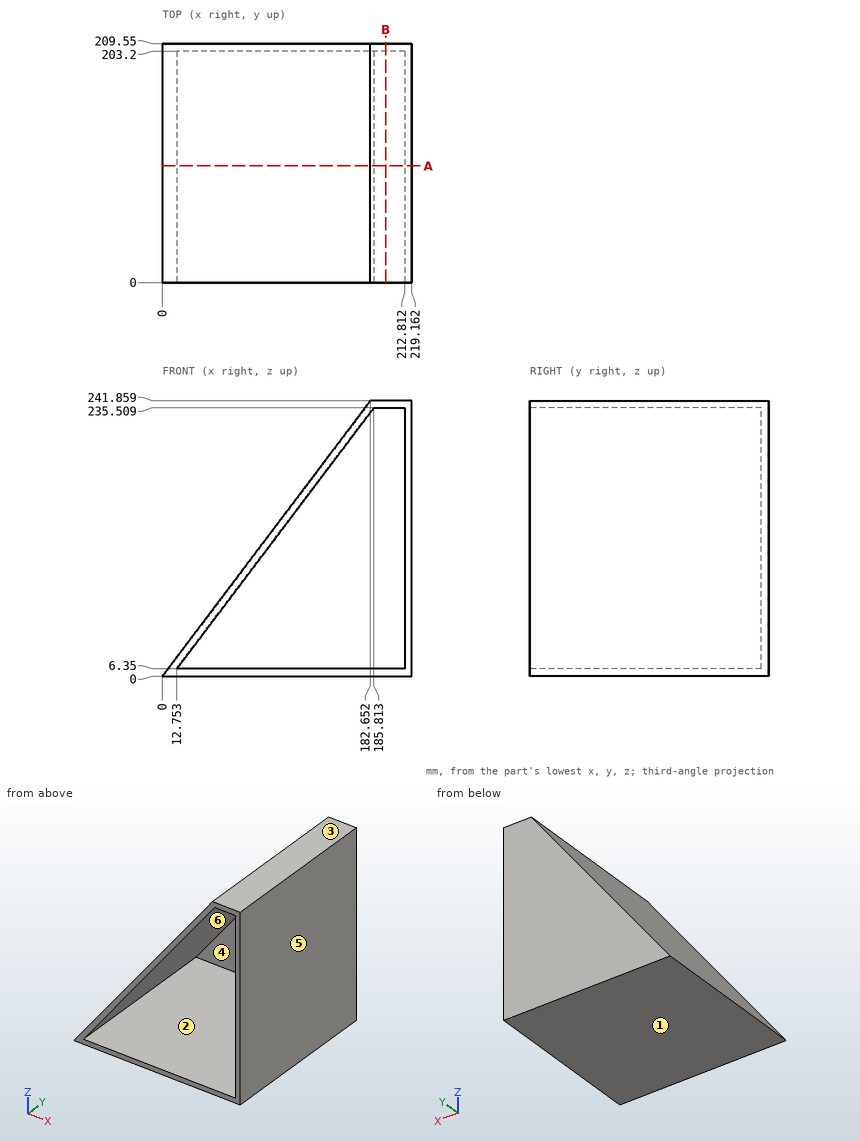
Geometry: see drawing. Coordinates: mm, zero at the bounding-box minimum. A direction names the side the tool comes from. Round coordinates to 2 decimals unless told otherwise and drop trailing zeros. Loops run counter-clockwise (first coordinate to the right, second up) from the corner with the lowest first, then second, coordinate; pieces in that order, holes last.
(1) Pull-direction query (X, two-part tool) for the marked faces 3, 4, 5 and 6; classes: +X half, -X half, draft (parallel to the pull), parting line (faces both ways), or undercut.
From the geometry:
face 3: draft
face 4: undercut
face 5: +X half
face 6: undercut
(2) Section query B-B (x = 196). Output: boundary loops of the cut face in (y, z), and give its area (3 significant figures).
From the geometry:
outline: (0, 0) - (209.55, 0) - (209.55, 241.86) - (0, 241.86) - (0, 235.51) - (203.2, 235.51) - (203.2, 6.35) - (0, 6.35) - close
area: 4,120 mm2
(3) Section query A-A (y = 102.5). Output: boundary loops of the cut face in (x, z), and give its area (3 significant figures).
From the geometry:
outline: (0, 0) - (219.16, 0) - (219.16, 241.86) - (182.65, 241.86) - close; hole (12.75, 6.35) - (212.81, 6.35) - (212.81, 235.51) - (185.81, 235.51) - close
area: 4,900 mm2
(4) Material intervals for probe 1 along Z at (x, y) = (202, 26); probe 2 along Y at (x, z) = (182, 51); probe 3 along X at (y, z) = (94, 57.5) (1 decimal), sorted ascending.
From the geometry:
probe 1: z = 0 to 6.35, 235.51 to 241.86
probe 2: y = 203.2 to 209.55
probe 3: x = 43.4 to 51.4, 212.8 to 219.2
(5) Access query for the marked faces 1 and 2. Directions: +Z, -Z, +X, -X, +Y, -Y. A direction counts if a zero-diameter tool reaches every point of the face in a straight line with its end or side. Return the directions, or none.
From the geometry:
face 1: -Z, +X, -X, +Y, -Y
face 2: -Y
(6) Contact query for flat-ended pins moving along their axis: pin 1 Ø6 at (x, y) = (129, 99) entering from +Z; pin 2 Ø10 at (x, y) = (81, 45.5) entering from +Z; pin 3 Ø3 at (x, y) = (152.5, 41.5) entering from +Z. Output: stop coordinate, or through.
From the geometry:
pin 1: stops at z = 174.79
pin 2: stops at z = 113.88
pin 3: stops at z = 203.92
